CAD build for the part. Positions are in the model's coordinates, mm. A direction names the side the tool comes from. Round coordinates to 2 decimals unless told otherwise and drop trailing zeros. Order: outer loops, then holes, each group sorted by start corner. A loop starts at its lowest first (then second) coordinate and runs counter-clockwise, first axis right, second up. Notation, with made-up numbers: (25, 28) - (52, 28) arc R16 ccw to (52, 43) - close; hole circle Ø11 at (35.5, -9.5). An arc over 180 degrees is marked (long way). Use one line per item in the form item = value. Start each with the question number.
from build123d import *

# Parameters (mm, degrees)
EXTRUDE_4_DEPTH = 32


with BuildPart() as part:
    # Эскиз1 → Бобышка-Вытянуть4 (new body)
    with BuildSketch(Plane.XY):
        with BuildLine():
            Line((4.299618531, 175.402841826), (4.299618531, 188.402841826))
            Line((4.299618531, 188.402841826), (84.299618531, 188.402841826))
            Line((84.299618531, 188.402841826), (84.299618531, 175.402841826))
            Line((84.299618531, 175.402841826), (84.299618531, 0))
            Line((84.299618531, 0), (84.299618531, -28))
            Line((84.299618531, -28), (0, -28))
            Line((0, -28), (0, 0))
            ThreePointArc((0, 0), (37.229295141, 21.561020186), (55.173142182, 60.662380285))
            ThreePointArc((55.173142182, 60.662380285), (56.797307883, 87.162380285), (55.173142182, 113.662380285))
            ThreePointArc((55.173142182, 113.662380285), (38.726552267, 151.940422917), (4.299618531, 175.402841826))
        make_face()
    extrude(amount=EXTRUDE_4_DEPTH)


solid = part.part
(1) Wall check: line 1 (Y direction, x = 47, z = 4); line 2 (Y direction, x = 37.5, z = 9); line 3 (X direction, y = 64, z = 10). Give the ranges that are in metal, low to high. Write a range as [from, to].
(2) Slice it at B-B (x = 50). Give the cut face in (y, z), and give its area (3 significant figures).
(3) Slice it at D-D (y = 28.5). Give the cut face in (x, z), and give its area (3 significant figures).
(4) Slice it at C-C (x = 10.5). Give the cut face in (y, z), and give its area (3 significant figures).
(5) Slice it at A-A (z = 12). Give the cut face in (x, y), and give its area (3 significant figures).
(6) Flat gauge pins, fed straight in: P1, Ø6.5, axis at y = 183, z = 8.5, coming from the -X side; P2, Ø12, axis at y = 156, z = 15, coming from the -X side. Where does each tip first touch, or does it go through?
(7) Which spindle directions (+Z, -Z, +X, -X, +Y, -Y) get a long thin tool onto all of the face, cutting with end or side? Do faces 1 (the flat face through (61, 82, 32)), 2 (the flat face through (4.3, 182, 16)), 3 (the cylindrical face through (39.101, 151.483, 15.776)). Say none if no direction does.
Results list:
q1.line_1 = [-28, 35.27], [139.56, 188.4]
q1.line_2 = [-28, 21.86], [153.39, 188.4]
q1.line_3 = [55.56, 84.3]
q2.outline = (-28, 0) - (41.45, 0) - (41.45, 32) - (-28, 32) - close; (133.22, 0) - (188.4, 0) - (188.4, 32) - (133.22, 32) - close
q2.area = 3,990 mm²
q3.outline = (42.79, 0) - (84.3, 0) - (84.3, 32) - (42.79, 32) - close
q3.area = 1,330 mm²
q4.outline = (-28, 0) - (3.18, 0) - (3.18, 32) - (-28, 32) - close; (173.07, 0) - (188.4, 0) - (188.4, 32) - (173.07, 32) - close
q4.area = 1,490 mm²
q5.outline = (0, -28) - (84.3, -28) - (84.3, 188.4) - (4.3, 188.4) - (4.3, 175.4) arc R74.5 cw to (55.17, 113.66) arc R217 cw to (55.17, 60.66) arc R71 cw to (0, 0) - close
q5.area = 10,300 mm²
q6.P1 = 4.3
q6.P2 = 28.68
q7.face_1 = +Z, +X, -X, +Y, -Y
q7.face_2 = +Z, -Z, -X, +Y
q7.face_3 = +Z, -Z, -X
